The model under review builds one solid part; all positions refer to its coordinate system, in mm. A direction names the side the tool comes from. Coordinates: 2 decimals unless noted, no trailing zeros. Loops run counter-clockwise (first coordinate to the right, second up) from the corner with the lowest first, then second, coordinate; pieces in that order, holes last. Notation, with made-up numbers: (38.5, 15) - (55.5, 15) arc R24 ccw to (55.5, 27) - close; hole circle Ø7 at (-6, 19). An arc over 180 degrees is marked (long way). Answer in a Markdown table with one row per item. Add a question column.
(1) We need section B-B on z = 0. Write out the cut boundary in (x, y), plus the area to 3 significant figures.
(2) We need section A-A on y = 0. Write out the cut boundary in (x, z), plus the area to 3 significant figures.
(3) We need section C-C on x = 2. Write out the cut boundary in (y, z), plus the area to 3 significant figures.
(4) For P1, Ø2, axis at x = 5, z = -0.5, coming from the -Y side; P2, Ø1.3, axis at y = 0, z = -0.5, coming from the +X side; P3, Ø1, axis at x = 5, z = -2, coming from the +Y side, all flat-tipped, find the tip position at first contact; note any pin that passes through.
(5) Machinability: for faces 1 (the flat face through (6.383, 3, 0)), 2 (the cylindrical face through (-3, -3, 0)), 3 (the flat face through (4.483, 0, 0)), which of the approach directions +Z, -Z, +X, -X, +Y, -Y give a long, thin tool a straight path to every point of the face, cutting with its end or side? Answer none if there is none.
(6) For line 1 along X through (y, z) = (-0.5, -1); line 2 along Y through (x, z) = (1.25, -0.25); line 3 along Y through (x, z) = (-5.5, 2.75), list the stretches that pass through material, from the lowest coordinate up.
from build123d import *

# Parameters (mm, degrees)
SKETCH2_W          = 1.9
SKETCH2_H          = 1.6
CUT_EXTRUDE1_DEPTH = 50


with BuildPart() as part:
    # Sketch1 → Revolve1 (revolve)
    with BuildSketch(Plane.XY):
        Polygon((6.382934587, 0), (6.382934587, 6), (3.382934587, 3), (-8.909958632, 3), (-9.617065413, 2.292893219), (-9.617065413, 0), align=None)
    revolve(axis=Axis((-31.290557053, 0, 0), (1, 0, 0)))

    # Sketch2 → Cut-Extrude1 (cut, symmetric)
    with BuildSketch(Plane.XY):
        with Locations((5.432934587, 0)):
            Rectangle(SKETCH2_W, SKETCH2_H)
    extrude(amount=CUT_EXTRUDE1_DEPTH, both=True, mode=Mode.SUBTRACT)


solid = part.part
Outcome:
| question | item | result |
|---|---|---|
| 1 | outline | (-9.62, -2.29) - (-8.91, -3) - (3.38, -3) - (6.38, -6) - (6.38, -0.8) - (4.48, -0.8) - (4.48, 0.8) - (6.38, 0.8) - (6.38, 6) - (3.38, 3) - (-8.91, 3) - (-9.62, 2.29) - close |
| 1 | area | 101 mm² |
| 2 | outline | (-9.62, -2.29) - (-8.91, -3) - (3.38, -3) - (4.48, -4.1) - (4.48, 4.1) - (3.38, 3) - (-8.91, 3) - (-9.62, 2.29) - close |
| 2 | area | 85.3 mm² |
| 3 | outline | circle Ø6 at (0, 0) |
| 3 | area | 28.3 mm² |
| 4 | P1 | y = -5.6 |
| 4 | P2 | x = 4.48 |
| 4 | P3 | y = 4.75 |
| 5 | face 1 | +Z, -Z, +X, +Y, -Y |
| 5 | face 2 | -X |
| 5 | face 3 | +Z, -Z, +X |
| 6 | line 1 | -9.62 to 4.48 |
| 6 | line 2 | -2.99 to 2.99 |
| 6 | line 3 | -1.2 to 1.2 |
